Here's how the part is built. I have some questions about the finished solid (model axes, mm). Give positions to 0.01 mm unless a question says otherwise; leave off trailing zeros. Write each loop counter-clockwise with the first axis right and the second up, starting at its lowest first coordinate (ties: lowest second). Pieces come first, ordered by that corner, then holes. Notation, with made-up numbers: (45.5, -2.5) - (102.5, -2.5) arc R15 ccw to (102.5, 19.5) - close; hole circle Ø7 at (33, -36.75). An arc over 180 degrees is marked (long way). One line per item, written item: value. Start each with the question number.
1) I'm going to push flat-ended pins straight in: P1, Ø1, axis at x = -18.5, z = 1.5, coming from the +Y side; P2, Ø1.5, axis at x = 8, z = 0.5, coming from the -Y side; P3, Ø1.6, axis at y = -35, z = 1, coming from the +X side. Where does each tip first touch, or does it pass through?
2) Imagine slicing it at C-C on z = 1.25. Write out the boundary of the cut face in (x, y).
3) Imagine slicing it at D-D on y = -14.5. Write out the boundary of the cut face in (x, z) (3 decimals).
4) Please list where these lines run through material, in increasing order: L1, parallel to Y at x = -25, z = 0.95; L2, parallel to Y at x = -12.5, z = 2.2; L3, parallel to X at y = -38.5, z = 2.8. Write a range as [from, to].
5) Imagine slicing it at A-A on y = 0. Write out the boundary of the cut face in (x, z) (3 decimals).
6) Imagine slicing it at B-B on x = -25. Write out the boundary of the cut face in (y, z) (3 decimals), plus the area to 3 significant figures.
from build123d import *

# Parameters (mm, degrees)
BOSS_EXTRUDE1_DEPTH = 3.175
FILLET1_R           = 7
FILLET2_R           = 5
SKETCH2_R           = 2.38125
CUT_EXTRUDE1_DEPTH  = 66.810946088
LPATTERN1_COUNT     = 3
LPATTERN1_PITCH     = 12.5


with BuildPart() as part:
    # Sketch1 → Boss-Extrude1 (new body)
    with BuildSketch(Plane.XY):
        with BuildLine():
            Line((-11.618950039, 11), (-36, 11))
            Line((-36, 11), (-36, -44))
            ThreePointArc((-36, -44), (-25, -55), (-14, -44))
            Line((-14, -44), (-14, -11))
            Line((-14, -11), (-11.618950039, -11))
            ThreePointArc((-11.618950039, -11), (16, 0), (-11.618950039, 11))
        make_face()
    extrude(amount=BOSS_EXTRUDE1_DEPTH)

    # Fillet1
    fillet1_edges = [part.edges().sort_by_distance(p)[0] for p in [
        (-36, 11, 1.5875),
    ]]
    fillet(fillet1_edges, radius=FILLET1_R)

    # Fillet2
    # the kernel refuses this fillet: 5 mm, written as the material it adds along each edge
    with BuildSketch(Plane(origin=(-14, -11, 0), x_dir=(1, 0, 0), z_dir=(0, 0, 1))) as fillet2_piece_1:
        with BuildLine():
            CenterArc((5, -4.259237102), FILLET2_R, 121.586822832, 58.413177168)
            Line((0, -4.259237102), (-0.1, -4.259237102))
            Line((-0.1, -4.259237102), (-0.1, 0))
            Line((-0.1, 0), (0, 0.1))
            ThreePointArc((0, 0.1), (1.190524981, 0.1), (2.328670961, 0.085184742))
            Line((2.328670961, 0.085184742), (2.381049961, 0))
        make_face()
    extrude(amount=3.175)

    # Sketch2 → Cut-Extrude1 (cut, through all)
    with BuildSketch(Plane.XY.offset(3.175)):
        Circle(SKETCH2_R)
    cut_extrude1 = extrude(amount=-CUT_EXTRUDE1_DEPTH, mode=Mode.SUBTRACT)

    # LPattern1: Cut-Extrude1 ×3
    with Locations(*[(-i * LPATTERN1_PITCH, 0, 0) for i in range(1, LPATTERN1_COUNT)]):
        add(cut_extrude1, mode=Mode.SUBTRACT)


solid = part.part
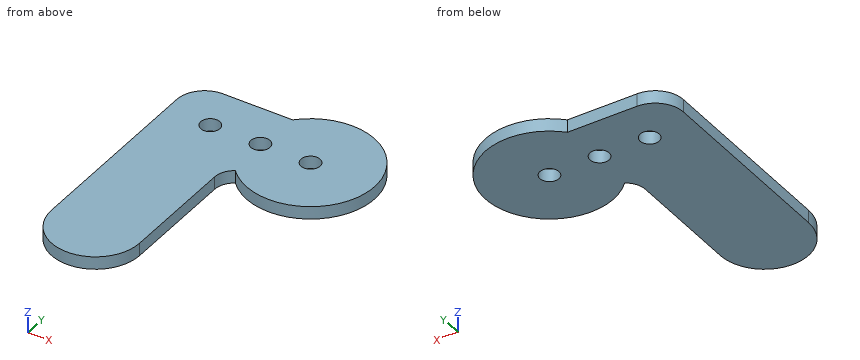
Numbers:
1. P1: y = 11
1. P2: y = -14.26
1. P3: x = -14
2. outline: (-36, -44) arc R11 ccw to (-14, -44) - (-14, -15.26) arc R5 cw to (-11.62, -11) arc R16 ccw (long way) to (-11.62, 11) - (-29, 11) arc R7 ccw to (-36, 4) - close; hole circle Ø4.76 at (-25, 0); hole circle Ø4.76 at (-12.5, 0); hole circle Ø4.76 at (0, 0)
3. outline: (-36, 0) - (-13.942, 0) - (-13.942, 3.175) - (-36, 3.175) - close; (-6.764, 0) - (6.764, 0) - (6.764, 3.175) - (-6.764, 3.175) - close
4. L1: [-55, -2.38], [2.38, 11]
4. L2: [-11.69, -2.38], [2.38, 11]
4. L3: [-36, -14]
5. outline: (-36, 0) - (-27.381, 0) - (-27.381, 3.175) - (-36, 3.175) - close; (-22.619, 0) - (-14.881, 0) - (-14.881, 3.175) - (-22.619, 3.175) - close; (-10.119, 0) - (-2.381, 0) - (-2.381, 3.175) - (-10.119, 3.175) - close; (2.381, 0) - (16, 0) - (16, 3.175) - (2.381, 3.175) - close
6. outline: (-55, 0) - (-2.381, 0) - (-2.381, 3.175) - (-55, 3.175) - close; (2.381, 0) - (11, 0) - (11, 3.175) - (2.381, 3.175) - close
6. area: 194 mm^2
